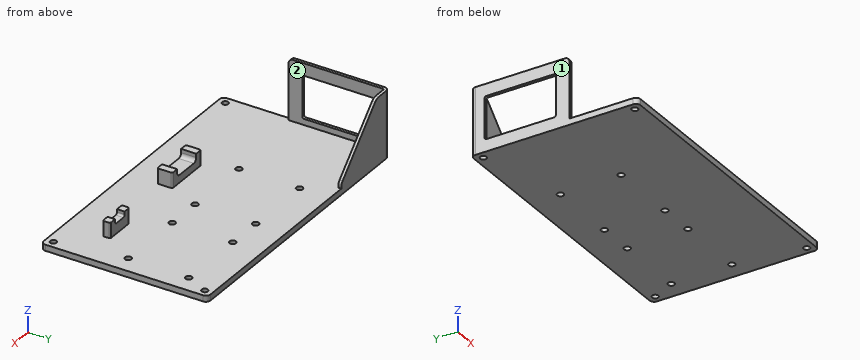
```python
from build123d import *

# Parameters (mm, degrees)
SKETCH_W        = 190
SKETCH_H        = 110
SKETCH_R        = 2.125
PAD_DEPTH       = 4
PAD001_DEPTH    = 40
SKETCH002_R     = 2.05
POCKET_DEPTH    = 4.001
SKETCH003_W     = 30
SKETCH003_H     = 10
SKETCH003_W_2   = 20
SKETCH003_H_2   = 5
PAD002_DEPTH    = 10
POCKET001_DEPTH = 30.001
SKETCH005_W     = 47
SKETCH005_H     = 28
POCKET002_DEPTH = 5
FILLET_R        = 1
FILLET001_R     = 3
FILLET002_R     = 1
FILLET003_R     = 3
CHAMFER_SIZE    = 37
FILLET004_R     = 5
FILLET005_R     = 1


with BuildPart() as part:
    # Sketch → Pad (new body)
    with BuildSketch(Plane.XY):
        Rectangle(SKETCH_W, SKETCH_H)
        with Locations((-33, 35)):
            Circle(SKETCH_R, mode=Mode.SUBTRACT)
        with Locations((-33, -5)):
            Circle(SKETCH_R, mode=Mode.SUBTRACT)
        with Locations((13, -5)):
            Circle(SKETCH_R, mode=Mode.SUBTRACT)
        with Locations((13, 35)):
            Circle(SKETCH_R, mode=Mode.SUBTRACT)
        with Locations((37, 35)):
            Circle(SKETCH_R, mode=Mode.SUBTRACT)
        with Locations((37, -5)):
            Circle(SKETCH_R, mode=Mode.SUBTRACT)
        with Locations((83, -5)):
            Circle(SKETCH_R, mode=Mode.SUBTRACT)
        with Locations((83, 35)):
            Circle(SKETCH_R, mode=Mode.SUBTRACT)
    extrude(amount=PAD_DEPTH)

    # Sketch001 (on Face14 of Pad) → Pad001 (join)
    with BuildSketch(Plane.XY.offset(4)):
        Polygon((-95, -10), (-95, 55), (-45, 55), (-45, 53), (-93, 53), (-93, -10), align=None)
    extrude(amount=PAD001_DEPTH)

    # Sketch002 (on Face6 of Pad001) → Pocket (cut, through all)
    with BuildSketch(Plane.XY.offset(4)):
        with Locations((-90, 50)):
            Circle(SKETCH002_R)
        with Locations((-90, -50)):
            Circle(SKETCH002_R)
        with Locations((90, -50)):
            Circle(SKETCH002_R)
        with Locations((90, 50)):
            Circle(SKETCH002_R)
    extrude(amount=-POCKET_DEPTH, mode=Mode.SUBTRACT)

    # Sketch003 (on Face6 of Pocket) → Pad002 (join)
    with BuildSketch(Plane.XY.offset(4)):
        with Locations((-10, -30)):
            Rectangle(SKETCH003_W, SKETCH003_H)
        with Locations((60, -27.5)):
            Rectangle(SKETCH003_W_2, SKETCH003_H_2)
    extrude(amount=PAD002_DEPTH)

    # Sketch004 (on Face30 of Pad002) → Pocket001 (cut, through all)
    with BuildSketch(Plane(origin=(0, -25, 0), x_dir=(-1, 0, 0), z_dir=(0, 1, 0))):
        with BuildLine():
            Line((0, 14), (20, 14))
            Line((20, 14), (20, 11.5))
            ThreePointArc((17.5, 9), (19.267767, 9.732233), (20, 11.5))
            Line((2.5, 9), (17.5, 9))
            ThreePointArc((0, 11.5), (0.732233, 9.732233), (2.5, 9))
            Line((0, 14), (0, 11.5))
        make_face()
        with BuildLine():
            Line((-65, 14), (-55, 14))
            Line((-55, 12), (-55, 14))
            ThreePointArc((-56.25, 10.75), (-55.366117, 11.116117), (-55, 12))
            Line((-63.75, 10.75), (-56.25, 10.75))
            ThreePointArc((-65, 12), (-64.633883, 11.116117), (-63.75, 10.75))
            Line((-65, 12), (-65, 14))
        make_face()
    extrude(amount=-POCKET001_DEPTH, mode=Mode.SUBTRACT)

    # Sketch005 (on Face8 of Pocket001) → Pocket002 (cut)
    with BuildSketch(Plane(origin=(-95, 0, 0), x_dir=(0, -1, 0), z_dir=(-1, 0, 0))):
        with Locations((-22.5, 22)):
            Rectangle(SKETCH005_W, SKETCH005_H)
    extrude(amount=-POCKET002_DEPTH, mode=Mode.SUBTRACT)

    # Fillet
    fillet_edges = [part.edges().sort_by_distance(p)[0] for p in [
        (-93, 53, 24),
    ]]
    fillet(fillet_edges, radius=FILLET_R)

    # Fillet001
    fillet001_edges = [part.edges().sort_by_distance(p)[0] for p in [
        (-95, 55, 24),
        (-95, -55, 2),
        (95, -55, 2),
        (95, 55, 2),
    ]]
    fillet(fillet001_edges, radius=FILLET001_R)

    # Fillet002
    fillet002_edges = [part.edges().sort_by_distance(p)[0] for p in [
        (-25, -25, 9),
        (-25, -35, 9),
        (5, -35, 9),
        (50, -25, 9),
        (50, -30, 9),
        (70, -30, 9),
        (70, -25, 9),
        (5, -25, 9),
    ]]
    fillet(fillet002_edges, radius=FILLET002_R)

    # Fillet003
    fillet003_edges = [part.edges().sort_by_distance(p)[0] for p in [
        (-94, -10, 44),
    ]]
    fillet(fillet003_edges, radius=FILLET003_R)

    # Chamfer
    chamfer_edges = [part.edges().sort_by_distance(p)[0] for p in [
        (-45, 54, 44),
    ]]
    chamfer(chamfer_edges, length=CHAMFER_SIZE)

    # Fillet004
    fillet004_edges = [part.edges().sort_by_distance(p)[0] for p in [
        (-45, 54, 7),
        (-82, 54, 44),
    ]]
    fillet(fillet004_edges, radius=FILLET004_R)

    # Fillet005
    fillet005_edges = [part.edges().sort_by_distance(p)[0] for p in [
        (-94, 46, 8),
        (-94, 46, 36),
        (-94, -1, 36),
        (-94, -1, 8),
    ]]
    fillet(fillet005_edges, radius=FILLET005_R)


solid = part.part
```
Check sheet for the modelled part. Datum: model origin and axes. Units: mm. Face numbers are marked on the shaded views. A direction names the side the tool comes from. Round coordinates to 2 decimals unless told otherwise and drop trailing zeros. Write each loop counter-clockwise with the first axis right and the second up, starting at its lowest first coordinate (ties: lowest second). Pieces come first, ordered by that corner, then holes. Notation, with made-up numbers: (7.5, 49) -> (47.5, 49) arc R12 ccw to (47.5, 66) -> close; hole circle Ø6 at (79.25, -5). An arc over 180 degrees is marked (long way). Put each result on its own line as item: value.
(1) Sectioned sample at A-A (z = 25). Enter the section's corners in (x, y), plus the area to 3 significant figures.
Values found:
outline: (-95, -10) -> (-93, -10) -> (-93, -1) -> (-95, -1) -> close; (-95, 46) -> (-93, 46) -> (-93, 52) arc R1 cw to (-92, 53) -> (-63, 53) -> (-63, 55) -> (-92, 55) arc R3 ccw to (-95, 52) -> close
area: 94.3 mm^2
(2) Sectioned sample at D-D (z = 39). Enter the section's corners in (x, y), plus the area to 3 significant figures.
Values found:
outline: (-95, -10) -> (-93, -10) -> (-93, 52) arc R1 cw to (-92, 53) -> (-77, 53) -> (-77, 55) -> (-92, 55) arc R3 ccw to (-95, 52) -> close
area: 160 mm^2
(3) Sectioned sample at C-C (x = 37). Enter the section's corners in (y, z) (3 decimals).
Values found:
outline: (-55, 0) -> (-7.125, 0) -> (-7.125, 4) -> (-55, 4) -> close; (-2.875, 0) -> (32.875, 0) -> (32.875, 4) -> (-2.875, 4) -> close; (37.125, 0) -> (55, 0) -> (55, 4) -> (37.125, 4) -> close
(4) Material ranges on line 1 (Y direction, x = 83, z = 3.1) (3 decimals); line 2 (Y direction, x = -66, z = 11); line 3 (Z direction, x = -19.5, y = 36.5), recorded low to high.
Values found:
line 1: y = -55 to -7.125, -2.875 to 32.875, 37.125 to 55
line 2: y = 53 to 55
line 3: z = 0 to 4
(5) Sectioned sample at B-B (y = 35). Enter the section's corners in (x, z) (3 decimals).
Values found:
outline: (-95, 0) -> (-35.125, 0) -> (-35.125, 4) -> (-93, 4) -> (-93, 8) -> (-95, 8) -> close; (-95, 36) -> (-93, 36) -> (-93, 44) -> (-95, 44) -> close; (-30.875, 0) -> (10.875, 0) -> (10.875, 4) -> (-30.875, 4) -> close; (15.125, 0) -> (34.875, 0) -> (34.875, 4) -> (15.125, 4) -> close; (39.125, 0) -> (80.875, 0) -> (80.875, 4) -> (39.125, 4) -> close; (85.125, 0) -> (95, 0) -> (95, 4) -> (85.125, 4) -> close
(6) Tool access check on the marked faces 1 and 2. Record the directions out of +Z, -Z, +X, -X, +Y, -Y that give a thin tool (end or side, any length) a straight path to the whole face; none if there is none.
Values found:
face 1: +Z, -Z, -X, +Y, -Y
face 2: +Z, +X, -Y
(7) Go/stop test with flat-tipped pins: pin 1 Ø6 at (x, y) = (42.5, 27.5) entering from -Z; pin 2 Ø3.5 at (x, y) = (90, -50) entering from +Z; pin 3 Ø4 at (x, y) = (-22, -32) entering from +Z; pin 4 Ø2.5 at (y, z) = (-27, 10) entering from +X. Record where each tip stops, or that it passes through.
Values found:
pin 1: stops at z = 0
pin 2: passes through
pin 3: stops at z = 14
pin 4: stops at x = 70
